Verification items for the finished model (mm, model axes). Give positions to 0.01 mm unless a question says otherwise; leave off trailing zeros. Write each loop counter-clockwise with the first axis right and the second up, starting at its lowest first coordinate (ties: lowest second). Pieces come first, ordered by that corner, then holes. Notation, with made-up numbers: M 41.5,46.5 L 73.5,46.5 A22 cw 73.5,56.5 Z; hole C 26,-11 d8. An arc over 180 degrees is marked long. Answer as a JSON object with one key per item and string values.
```python
from build123d import *

# Parameters (mm, degrees)
F0_W      = 1270
F0_H      = 1270
F1_DEPTH  = 1.5875
F2_W      = 736.6
F2_H      = 723.9
F3_DEPTH  = 3.176
F2_W_2    = 347.218
F2_H_2    = 889
F4_DEPTH  = 3.176
F2_H_3    = 127
F5_DEPTH  = 3.176
F6_DEPTH  = 3.176
F7_DEPTH  = 3.176
F2_W_3    = 423.164
F2_H_4    = 431.8
F8_DEPTH  = 3.176
F9_DEPTH  = 3.176
F10_DEPTH = 3.176


with BuildPart() as f1:
    # F0 (on Front) → F1 (new body, symmetric)
    with BuildSketch(Plane.XZ):
        with Locations((-0.489235, 87.176618)):
            Rectangle(F0_W, F0_H)
    extrude(amount=F1_DEPTH, both=True)

    # F2 (on face) → F3 (cut, through all)
    with BuildSketch(Plane.XZ.offset(1.5875)):
        with Locations((-229.089235, 284.026618)):
            Rectangle(F2_W, F2_H)
    extrude(amount=-F3_DEPTH, mode=Mode.SUBTRACT)

    # F2 (on face) → F4 (cut, through all)
    with BuildSketch(Plane.XZ.offset(1.5875)):
        with Locations((422.801765, 201.476618)):
            Rectangle(F2_W_2, F2_H_2)
    extrude(amount=-F4_DEPTH, mode=Mode.SUBTRACT)

    # F2 (on face) → F5 (cut, through all)
    with BuildSketch(Plane.XZ.offset(1.5875)):
        with Locations((-423.780235, -179.523382)):
            Rectangle(F2_W_2, F2_H_3)
    extrude(amount=-F5_DEPTH, mode=Mode.SUBTRACT)

    # F2 (on face) → F6 (cut, through all)
    with BuildSketch(Plane.XZ.offset(1.5875)):
        with Locations((-423.780235, -319.223382)):
            Rectangle(F2_W_2, F2_H_3)
    extrude(amount=-F6_DEPTH, mode=Mode.SUBTRACT)

    # F2 (on face) → F7 (cut, through all)
    with BuildSketch(Plane.XZ.offset(1.5875)):
        with Locations((-423.780235, -460.295247)):
            Rectangle(F2_W_2, F2_H_3)
    extrude(amount=-F7_DEPTH, mode=Mode.SUBTRACT)

    # F2 (on face) → F8 (cut, through all)
    with BuildSketch(Plane.XZ.offset(1.5875)):
        with Locations((-0.489235, -331.923382)):
            Rectangle(F2_W_3, F2_H_4)
    extrude(amount=-F8_DEPTH, mode=Mode.SUBTRACT)

    # F2 (on face) → F9 (cut, through all)
    with BuildSketch(Plane.XZ.offset(1.5875)):
        with Locations((422.801765, -319.223382)):
            Rectangle(F2_W_2, F2_H_3)
    extrude(amount=-F9_DEPTH, mode=Mode.SUBTRACT)

    # F2 (on face) → F10 (cut, through all)
    with BuildSketch(Plane.XZ.offset(1.5875)):
        with Locations((422.801765, -460.295247)):
            Rectangle(F2_W_2, F2_H_3)
    extrude(amount=-F10_DEPTH, mode=Mode.SUBTRACT)


solid = f1.part
```
1) Section check A-A on x = -348.5. Record the boundary of the cut face in (y, z).
Completed:
{"outline": "M -1.59,-547.82 L 1.59,-547.82 L 1.59,-523.8 L -1.59,-523.8 Z; M -1.59,-396.8 L 1.59,-396.8 L 1.59,-382.72 L -1.59,-382.72 Z; M -1.59,-255.72 L 1.59,-255.72 L 1.59,-243.02 L -1.59,-243.02 Z; M -1.59,-116.02 L 1.59,-116.02 L 1.59,-77.92 L -1.59,-77.92 Z; M -1.59,645.98 L 1.59,645.98 L 1.59,722.18 L -1.59,722.18 Z"}
2) Section check B-B on z = 123. Record the boundary of the cut face in (x, y).
Completed:
{"outline": "M -635.49,-1.59 L -597.39,-1.59 L -597.39,1.59 L -635.49,1.59 Z; M 139.21,-1.59 L 249.19,-1.59 L 249.19,1.59 L 139.21,1.59 Z; M 596.41,-1.59 L 634.51,-1.59 L 634.51,1.59 L 596.41,1.59 Z"}
3) Section check C-C on x = -195. Record the boundary of the cut face in (y, z).
Completed:
{"outline": "M -1.59,-116.02 L 1.59,-116.02 L 1.59,-77.92 L -1.59,-77.92 Z; M -1.59,645.98 L 1.59,645.98 L 1.59,722.18 L -1.59,722.18 Z"}
4) Section check D-D on z = -158. Record the boundary of the cut face in (x, y).
Completed:
{"outline": "M -635.49,-1.59 L -597.39,-1.59 L -597.39,1.59 L -635.49,1.59 Z; M -250.17,-1.59 L -212.07,-1.59 L -212.07,1.59 L -250.17,1.59 Z; M 211.09,-1.59 L 249.19,-1.59 L 249.19,1.59 L 211.09,1.59 Z; M 596.41,-1.59 L 634.51,-1.59 L 634.51,1.59 L 596.41,1.59 Z"}
5) Go/stop test with a flat-tipped pin: pin 1 (5 mm diameter, centred on x = -316, z = -121, fed in from -Y). Record where the tip stops, or that it passes through.
Completed:
{"pin 1": "passes through"}
6) Thickness scan on L1, parallel to X at y = 1.5, z = 355.5; L2, parallel to Z at x = -421.5, y = -0.1; L3, parallel to Z at x = 436, y = 1. Record the ranges inside material, lowest first.
Completed:
{"L1": "x = -635.49 to -597.39, 139.21 to 249.19, 596.41 to 634.51", "L2": "z = -547.82 to -523.8, -396.8 to -382.72, -255.72 to -243.02, -116.02 to -77.92, 645.98 to 722.18", "L3": "z = -547.82 to -523.8, -396.8 to -382.72, -255.72 to -243.02, 645.98 to 722.18"}
